Verification items for this drawing (mm, ordinates from the low corner). A direction names the side the tool comes from. Coordinates: 2 decimals unless noted, no trailing zeros. Order: outer loops, then holes, each group sorted by start corner. A loop starts at its lowest first (then second) coordinate and runs counter-clockwise, first axis right, second up. Notation, with made-up numbers: (-32.75, 12) -> (4.25, 12) arc R21 ccw to (4.25, 26) -> close; hole circle Ø6 at (-39.5, 70). An arc over 180 degrees is marked (long way). Answer as CSV lines item,"result". Start each with the question number.
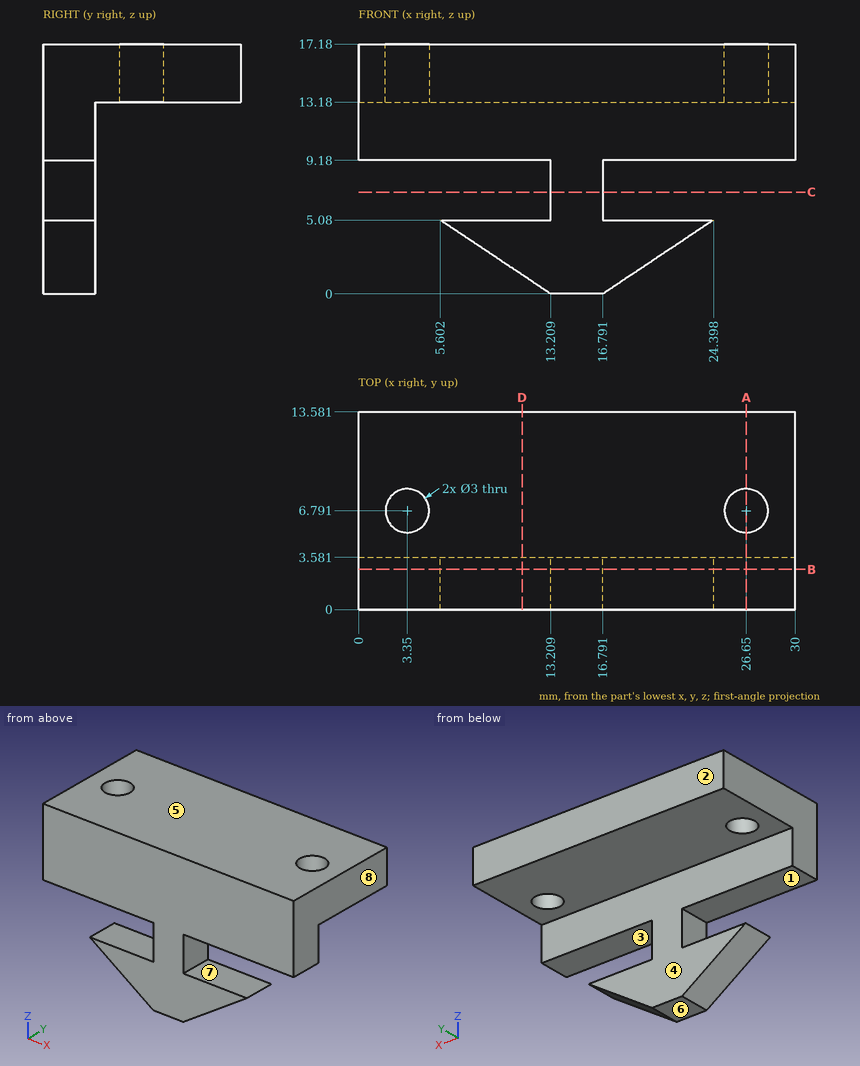
Q1. Release check for a two-part mould opening along Z. For the marked faces 6, 7 and 8 record: released by +Z, released by -Z, zero draft, split by the parting line, or undercut.
Q2. Go/stop test with flat-tipped pins: pin 1 Ø3 at (y, z) = (1.5, 7.5) entering from -X; pin 2 Ø3 at (x, y) = (23, 2.5) entering from -Z (1 decimal); pin 3 Ø6 at (x, z) = (17.5, 2.5) entering from +Y. Record where each tip stops, or that it passes through.
Q3. Sectioned sample at A-A, the plane x = 26.65. Record the cut outline in (y, z).
Q4. Sectioned sample at C-C, the plane z = 7. Record the cut outline in (x, y), then the cut area to 3 significant figures.
Q5. Thickness scan on L1, parallel to Y at x = 26.65, z = 15.95; L2, parallel to X at y = 5.75, z = 14.5; L3, parallel to Z at x = 10, y = 6.75. Record the ranges inside material, lowest first.
Q6. Sectioned sample at B-B, the plane y = 2.75. Record the cut outline in (x, z).
Q7. Sectioned sample at D-D, the plane x = 11.25. Record the cut outline in (y, z).
Q8. Access from +Z, -Z, +X, -X, +Y, -Y to the whole of each face (thin tool, end or side, straight path). Record for the marked faces 1, 2, 3, 4 and 5.
Geometry results:
1,face 6,"released by -Z"
1,face 7,"undercut"
1,face 8,"zero draft"
2,pin 1,"stops at x = 13.21"
2,pin 2,"stops at z = 3.1"
2,pin 3,"stops at y = 3.58"
3,outline,"(0, 9.18) -> (3.58, 9.18) -> (3.58, 13.18) -> (5.29, 13.18) -> (5.29, 17.18) -> (0, 17.18) -> close; (8.29, 13.18) -> (13.58, 13.18) -> (13.58, 17.18) -> (8.29, 17.18) -> close"
4,outline,"(13.21, 0) -> (16.79, 0) -> (16.79, 3.58) -> (13.21, 3.58) -> close"
4,area,"12.8 mm^2"
5,L1,"y = 0 to 5.29, 8.29 to 13.58"
5,L2,"x = 0 to 2.27, 4.43 to 25.57, 27.73 to 30"
5,L3,"z = 13.18 to 17.18"
6,outline,"(0, 9.18) -> (13.21, 9.18) -> (13.21, 5.08) -> (5.6, 5.08) -> (13.21, 0) -> (16.79, 0) -> (24.4, 5.08) -> (16.79, 5.08) -> (16.79, 9.18) -> (30, 9.18) -> (30, 17.18) -> (0, 17.18) -> close"
7,outline,"(0, 1.31) -> (3.58, 1.31) -> (3.58, 5.08) -> (0, 5.08) -> close; (0, 9.18) -> (3.58, 9.18) -> (3.58, 13.18) -> (13.58, 13.18) -> (13.58, 17.18) -> (0, 17.18) -> close"
8,face 1,"-X, +Y, -Y"
8,face 2,"+Z, -Z, +X, -X, +Y"
8,face 3,"+X, +Y, -Y"
8,face 4,"-Z, +X, -X, +Y"
8,face 5,"+Z, +X, -X, +Y, -Y"
